Check sheet for the modelled part. Datum: model origin and axes. Units: mm. Face numbers are marked on the shaded views. A direction names the side the tool comes from. Round coordinates to 2 decimals unless told otherwise and drop trailing zeros. Loops run counter-clockwise (first coordinate to the right, second up) from the corner with the lowest first, then second, coordinate; pieces in that order, holes last. Notation, with made-up numbers: (32.25, 69.5) -> (67.25, 69.5) arc R20 cw to (67.25, 76.5) -> close; hole circle Ø2 at (-35.5, 87). An arc over 180 degrees is marked (long way). Return JSON: item names as keys, results as strings.
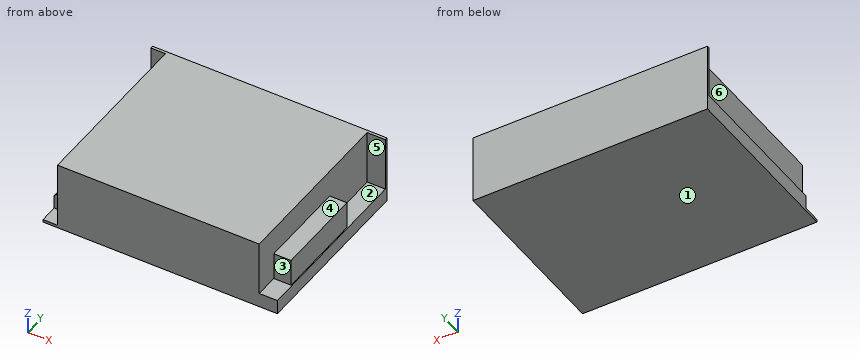
from build123d import *

# Parameters (mm, degrees)
SKETCH_1_W          = 129
SKETCH_1_H          = 98
EXTRUDE_1_DEPTH     = 38
SKETCH_2_W          = 10
SKETCH_2_H          = 96.5
CUT_EXTRUDE_1_DEPTH = 30
SKETCH_3_W          = 9.5
SKETCH_3_H          = 50
EXTRUDE_2_DEPTH     = 15
SKETCH_4_W          = 29
SKETCH_4_H          = 96.5
CUT_EXTRUDE_2_DEPTH = 8
CHAMFER_1_SIZE      = 8
CUT_EXTRUDE_3_DEPTH = 10


with BuildPart() as part:
    # 草图1 → 凸台-拉伸1 (new body)
    with BuildSketch(Plane.XY):
        with Locations((64.5, 49)):
            Rectangle(SKETCH_1_W, SKETCH_1_H)
    extrude(amount=EXTRUDE_1_DEPTH)

    # 草图2 → 切除-拉伸1 (cut)
    with BuildSketch(Plane.XY.offset(38)):
        with Locations((124, 48.25)):
            Rectangle(SKETCH_2_W, SKETCH_2_H)
    extrude(amount=-CUT_EXTRUDE_1_DEPTH, mode=Mode.SUBTRACT)

    # 草图3 → 凸台-拉伸2 (add)
    with BuildSketch(Plane.XY.offset(8)):
        with Locations((123.75, 38)):
            Rectangle(SKETCH_3_W, SKETCH_3_H)
    extrude(amount=EXTRUDE_2_DEPTH)

    # 草图4 → 切除-拉伸2 (cut)
    with BuildSketch(Plane.ZY):
        with Locations((23.5, 48.25)):
            Rectangle(SKETCH_4_W, SKETCH_4_H)
    extrude(amount=-CUT_EXTRUDE_2_DEPTH, mode=Mode.SUBTRACT)

    # 倒角1
    chamfer_1_edges = [part.edges().sort_by_distance(p)[0] for p in [
        (8, 48.25, 9),
    ]]
    chamfer(chamfer_1_edges, length=CHAMFER_1_SIZE - 0.0001)  # a hair under: the kernel refuses the full size

    # 草图5 → 切除-拉伸3 (cut)
    with BuildSketch(Plane.XZ):
        Polygon((0, 9), (8, 17), (8, 1.5), (0, 1.5), align=None)
    extrude(amount=-CUT_EXTRUDE_3_DEPTH, mode=Mode.SUBTRACT)


solid = part.part
Q1. Go/stop test with flat-tipped pins: pin 1 (4 mm diameter, centred on x = 4.5, z = 12, fed in from -Y); pin 2 (4 mm diameter, centred on y = 47.5, z = 19.5, fed in from -X); pin 3 (4 mm diameter, centred on x = 2.5, z = 19.5, fed in from -Y). Record where each tip stops, or that it passes through.
Results list:
{"pin 1": "y = 10", "pin 2": "x = 8", "pin 3": "y = 96.5"}
Q2. Material ranges on line 1 (X direction, y = 94, z = 17); line 2 (X direction, y = 56, z = 9), recorded low to high.
Results list:
{"line 1": "8 to 119", "line 2": "0 to 128.5"}
Q3. Tool access check on the marked faces 4, 5 and 6. Record the directions out of +Z, -Z, +X, -X, +Y, -Y that give a thin tool (end or side, any length) a straight path to the whole face; none if there is none.
Results list:
{"face 4": "+Z, +X, -Y", "face 5": "+Z, +X", "face 6": "+Z, -X, -Y"}
Q4. Section check D-D (z = 13.5). Record the boundary of the cut face in (x, y), then the cut area to 3 significant figures.
Results list:
{"outline": "(0, 96.5) -> (4.5, 96.5) -> (4.5, 10) -> (8, 10) -> (8, 0) -> (119, 0) -> (119, 13) -> (128.5, 13) -> (128.5, 63) -> (119, 63) -> (119, 96.5) -> (129, 96.5) -> (129, 98) -> (0, 98) -> close", "area": "11,700 mm^2"}
Q5. Draft check along Y on the marked faces 1, 2 and 3. Enter one of: released by +Y, released by -Y, zero draft, split by the parting line, or undercut.
Results list:
{"face 1": "zero draft", "face 2": "undercut", "face 3": "released by -Y"}
Q6. Section check A-A (z = 34.5). Record the boundary of the cut face in (x, y).
Results list:
{"outline": "(0, 96.5) -> (8, 96.5) -> (8, 0) -> (119, 0) -> (119, 96.5) -> (129, 96.5) -> (129, 98) -> (0, 98) -> close"}
